Input: part model. Units: mm. Frame: model coordinates. A direction names the side the tool comes from. Give positions to 0.01 mm unless a question says otherwise; leave off trailing zeros. Loops run counter-clockwise (first coordinate to the right, second up) from the corner with the lowest first, then second, coordinate; pieces in that order, holes last. Notation, with made-up numbers: M 7.5,-15.75 L 30.5,-15.75 A19 ccw 30.5,2.25 Z; hole C 76,-27 d5. An arc over 180 degrees is marked long. One line per item, written item: value. Start each with the question number.
(1) Section C-C on x = 18. Output: boundary loops of the cut face in (y, z), plus the area to 3 significant figures.
(2) Section A-A on x = -49.5. Output: boundary loops of the cut face in (y, z).
(3) Section D-D on z = 3.5. State how many separate pieces and enclosed holes the cut face has, plus the area to 3 significant figures.
(4) Pull-direction query (Y, two-part tool) for faces 1 (the flat face through (-70, 26, 2)), 2 (the cylindrical face through (-92.148, 17.057, 2.465)), 3 (the cylindrical face through (90.88, -16.99, 2.46)), 4 (the flat face through (-50, 20.064, 2)); classes: released by +Y, released by -Y, zero draft, split by the parting line, or undercut.
(5) Ray query, line 1 along Y through (x, z) = (18, 2.8); line 2 along X through (y, z) = (-24.5, 2.6); line 3 along Y through (x, z) = (11, 2). Return the intervals inside material, ascending. Write a range as from..to.
(6) Section B-B on y = -25. Output: boundary loops of the cut face in (x, z).
(7) Access query for faces 5 (the cylindrical face through (-40, 25, 2)), 6 (the flat face through (70, 26, 2)). Directions: +Z, -Z, +X, -X, +Y, -Y. A direction counts if a zero-diameter tool reaches every point of the face in a straight line with its end or side. Return the directions, or none.
```python
from build123d import *

# Parameters (mm, degrees)
SKETCH1_R           = 1.7
BOSS_EXTRUDE1_DEPTH = 5
CUT_EXTRUDE4_DEPTH  = 5
SKETCH3_R           = 1.6
SKETCH3_R_2         = 1.7
CUT_EXTRUDE7_DEPTH  = 5


with BuildPart() as part:
    # Sketch1 → Boss-Extrude1 (new body)
    with BuildSketch(Plane.XY):
        with BuildLine():
            Line((-60, 42.5), (60, 42.5))
            ThreePointArc((60, 42.5), (67.071067812, 39.571067812), (70, 32.5))
            Line((70, 32.5), (70, 20))
            Line((70, 20), (83.73, 20))
            ThreePointArc((83.73, 20), (90.801067812, 17.071067812), (93.73, 10))
            Line((93.73, 10), (93.73, -10))
            ThreePointArc((93.73, -10), (90.801067812, -17.071067812), (83.73, -20))
            Line((83.73, -20), (70, -20))
            Line((70, -20), (70, -32.5))
            ThreePointArc((70, -32.5), (67.071067812, -39.571067812), (60, -42.5))
            Line((60, -42.5), (-60, -42.5))
            ThreePointArc((-60, -42.5), (-67.071067812, -39.571067812), (-70, -32.5))
            Line((-70, -32.5), (-70, -19.935858434))
            Line((-70, -19.935858434), (-85, -19.935858434))
            ThreePointArc((-85, -19.935858434), (-92.071067812, -17.006926246), (-95, -9.935858434))
            Line((-95, -9.935858434), (-95, 10.064141566))
            ThreePointArc((-95, 10.064141566), (-92.071067812, 17.135209378), (-85, 20.064141566))
            Line((-85, 20.064141566), (-70, 20.064141566))
            Line((-70, 20.064141566), (-70, 32.5))
            ThreePointArc((-70, 32.5), (-67.071067812, 39.571067812), (-60, 42.5))
        make_face()
        with Locations((-87, 15)):
            Circle(SKETCH1_R, mode=Mode.SUBTRACT)
        with Locations((-62.5, 15)):
            Circle(SKETCH1_R, mode=Mode.SUBTRACT)
        with Locations((-62.5, -15)):
            Circle(SKETCH1_R, mode=Mode.SUBTRACT)
        with Locations((-87, -15)):
            Circle(SKETCH1_R, mode=Mode.SUBTRACT)
        with Locations((62.5, 15)):
            Circle(SKETCH1_R, mode=Mode.SUBTRACT)
        with Locations((62.5, -15)):
            Circle(SKETCH1_R, mode=Mode.SUBTRACT)
        with Locations((87, -15)):
            Circle(SKETCH1_R, mode=Mode.SUBTRACT)
        with Locations((87, 15)):
            Circle(SKETCH1_R, mode=Mode.SUBTRACT)
        with Locations((-60, 32.5)):
            Circle(SKETCH1_R, mode=Mode.SUBTRACT)
        with Locations((60, 32.5)):
            Circle(SKETCH1_R, mode=Mode.SUBTRACT)
        with Locations((60, -32.5)):
            Circle(SKETCH1_R, mode=Mode.SUBTRACT)
        with Locations((-60, -32.5)):
            Circle(SKETCH1_R, mode=Mode.SUBTRACT)
    extrude(amount=BOSS_EXTRUDE1_DEPTH)

    # Sketch2 → Cut-Extrude4 (cut)
    with BuildSketch(Plane.XY):
        with BuildLine():
            Line((20, 37.5), (-20, 37.5))
            ThreePointArc((-20, 37.5), (-25, 32.5), (-20, 27.5))
            Line((-20, 27.5), (20, 27.5))
            ThreePointArc((20, 27.5), (25, 32.5), (20, 37.5))
        make_face()
        with BuildLine():
            Line((20, -27.5), (-20, -27.5))
            ThreePointArc((-20, -27.5), (-25, -32.5), (-20, -37.5))
            Line((-20, -37.5), (20, -37.5))
            ThreePointArc((20, -37.5), (25, -32.5), (20, -27.5))
        make_face()
        with BuildLine():
            Line((-45, 30.064141566), (-55, 30.064141566))
            ThreePointArc((-55, 30.064141566), (-60, 25.064141566), (-55, 20.064141566))
            Line((-55, 20.064141566), (-45, 20.064141566))
            ThreePointArc((-45, 20.064141566), (-40, 25.064141566), (-45, 30.064141566))
        make_face()
        with BuildLine():
            Line((-45, -19.935858434), (-55, -19.935858434))
            ThreePointArc((-55, -19.935858434), (-60, -24.935858434), (-55, -29.935858434))
            Line((-55, -29.935858434), (-45, -29.935858434))
            ThreePointArc((-45, -29.935858434), (-40, -24.935858434), (-45, -19.935858434))
        make_face()
        with BuildLine():
            Line((53.73, 30), (43.73, 30))
            ThreePointArc((43.73, 30), (38.73, 25), (43.73, 20))
            Line((43.73, 20), (53.73, 20))
            ThreePointArc((53.73, 20), (58.73, 25), (53.73, 30))
        make_face()
        with BuildLine():
            Line((53.73, -20), (43.73, -20))
            ThreePointArc((43.73, -20), (38.73, -25), (43.73, -30))
            Line((43.73, -30), (53.73, -30))
            ThreePointArc((53.73, -30), (58.73, -25), (53.73, -20))
        make_face()
    extrude(amount=CUT_EXTRUDE4_DEPTH, mode=Mode.SUBTRACT)

    # Sketch3 → Cut-Extrude7 (cut)
    with BuildSketch(Plane.XY):
        with Locations((-23, -17.8)):
            Circle(SKETCH3_R)
        with Locations((-23, 18)):
            Circle(SKETCH3_R)
        with Locations((22.6, -18.168627451)):
            Circle(SKETCH3_R)
        with Locations((22.6, 18)):
            Circle(SKETCH3_R)
        with Locations((-18, 18)):
            Circle(SKETCH3_R_2)
        with Locations((18, -18)):
            Circle(SKETCH3_R_2)
        with Locations((-18, -18)):
            Circle(SKETCH3_R_2)
        with Locations((18, 18)):
            Circle(SKETCH3_R_2)
    extrude(amount=CUT_EXTRUDE7_DEPTH, mode=Mode.SUBTRACT)


solid = part.part
```
Output values:
1. outline: M -42.5,0 L -37.5,0 L -37.5,5 L -42.5,5 Z; M -27.5,0 L -19.7,0 L -19.7,5 L -27.5,5 Z; M -16.3,0 L 16.3,0 L 16.3,5 L -16.3,5 Z; M 19.7,0 L 27.5,0 L 27.5,5 L 19.7,5 Z; M 37.5,0 L 42.5,0 L 42.5,5 L 37.5,5 Z
1. area: 291 mm²
2. outline: M -42.5,0 L -29.94,0 L -29.94,5 L -42.5,5 Z; M -19.94,0 L 20.06,0 L 20.06,5 L -19.94,5 Z; M 30.06,0 L 42.5,0 L 42.5,5 L 30.06,5 Z
3. separate pieces: 1
3. enclosed holes: 26
3. area: 11,800 mm²
4. face 1: zero draft
4. face 2: released by +Y
4. face 3: released by -Y
4. face 4: undercut
5. line 1: y = -42.5..-37.5, -27.5..-19.7, -16.3..16.3, 19.7..27.5, 37.5..42.5
5. line 2: x = -70..-59.98, -40.02..38.76, 58.7..70
5. line 3: y = -42.5..-37.5, -27.5..27.5, 37.5..42.5
6. outline: M -70,0 L -60,0 L -60,5 L -70,5 Z; M -40,0 L 38.73,0 L 38.73,5 L -40,5 Z; M 58.73,0 L 70,0 L 70,5 L 58.73,5 Z
7. face 5: +Z, -Z
7. face 6: +Z, -Z, +X, +Y
